Work out the finished part from the listing and answer in its coordinate system (mm). Give positions to 0.01 mm unless a question says otherwise; leave off trailing zeros. Order: outer loops, then holes, each group sorted by start corner. A loop starts at its lowest first (then second) coordinate and runs counter-clockwise, first axis right, second up. Notation, with made-up numbers: (-39, 65.25) - (-28, 65.25) arc R11 cw to (-28, 73.25) - close; hole circle Ø9 at (-0.5, 41). An arc over 180 degrees is marked (long way). Write each question's results on one line, items separated by ' | '.
Autodesk Inventor part; units mm, degrees
ref_plane "YZ Plane" through (0, 0, 0) normal (1, 0, 0) x (0, 1, 0)
ref_plane "XZ Plane" through (0, 0, 0) normal (0, 1, 0) x (-1, 0, 0)
ref_plane "XY Plane" through (0, 0, 0) normal (0, 0, 1) x (1, 0, 0)
sketch "Sketch2" plane through (0, 0, 0) normal (0, 0, 1) x (1, 0, 0)
  circle A0 centre (0, 0) radius 6.35
  line L0 (0, 0) -> (0, 11.35)
  line L1 (0, 11.35) -> (9.8294, 5.675)
  line L2 (9.8294, 5.675) -> (9.8294, -5.675)
  line L3 (9.8294, -5.675) -> (0, -11.35)
  line L4 (0, -11.35) -> (-9.8294, -5.675)
  line L5 (-9.8294, -5.675) -> (-9.8294, 5.675)
  line L6 (-9.8294, 5.675) -> (0, 11.35)
  dimension "d11" = 12.7
extrude "Extrusion2" add sketch "Sketch2" along normal blind 30
thread "Thread2"
chamfer "Chamfer2" distance 1 angle 45 18 edges at (4.9147, 8.5125, 30) (9.8294, 0, 30) (4.9147, -8.5125, 30) (-4.9147, -8.5125, 30) (-9.8294, 0, 30) (-4.9147, 8.5125, 30) (9.8294, 5.675, 15) (9.8294, -5.675, 15) (0, -11.35, 15) (-9.8294, -5.675, 15) (-9.8294, 5.675, 15) (0, 11.35, 15) (-4.9147, 8.5125, 0) (4.9147, 8.5125, 0) (9.8294, 0, 0) (4.9147, -8.5125, 0) (-4.9147, -8.5125, 0) (-9.8294, 0, 0)
properties part number "5302_Brass_Nut_0.5_20_Tx_Rx_Relative_Positioning_MPSv2_v1" material "Brass, Soft Yellow"
1. A cutting plane is placed at B-B, the plane x = 6. Write down the section's boundary in (y, z), then the cut area to 3 significant figures.
Answer list:
outline: (-7.89, 1) - (-6.73, 0) - (-2.08, 0) - (-2.08, 30) - (-6.73, 30) - (-7.89, 29) - close; (2.08, 0) - (6.73, 0) - (7.89, 1) - (7.89, 29) - (6.73, 30) - (2.08, 30) - close | area: 346 mm^2
2. Straight lines are drawn through the part: line 1 (X direction, y = 0, z = 18); line 2 (Y direction, x = 0, z = 23.75); line 3 (Y direction, x = -4.25, z = 14). For each, find the intervals that lie inside material, in ascending order. Write a range as [from, to].
Answer list:
line 1: [-9.83, -6.35], [6.35, 9.83] | line 2: [-10.85, -6.35], [6.35, 10.85] | line 3: [-8.9, -4.72], [4.72, 8.9]
3. A cutting plane is placed at A-A, the plane y = 0. Write down the section's boundary in (x, z).
Answer list:
outline: (-9.83, 1) - (-8.83, 0) - (-6.35, 0) - (-6.35, 30) - (-8.83, 30) - (-9.83, 29) - close; (6.35, 0) - (8.83, 0) - (9.83, 1) - (9.83, 29) - (8.83, 30) - (6.35, 30) - close
4. A cutting plane is placed at D-D, the plane y = 7. Write down the section's boundary in (x, z).
Answer list:
outline: (-7.53, 1) - (-5.53, 0) - (5.53, 0) - (7.53, 1) - (7.53, 29) - (5.53, 30) - (-5.53, 30) - (-7.53, 29) - close
5. Given P1, Ø11.5, axis at x = 0, y = 0, coming from the +Z side; P2, Ø5, axis at y = 8.5, z = 7.5, coming from the +X side; P3, Ø4, axis at x = -6, z = 13, coming from the -Y side; P4, Ø3, axis at x = -7, z = 3.5, coming from the +Y side, each flat-ended and moving along its own axis, determine where each tip first touches the part or whether it passes through.
Answer list:
P1: through | P2: x = 9.06 | P3: y = -9.04 | P4: y = 8.17
6. A cutting plane is placed at C-C, the plane z = 7.5. Write down the section's boundary in (x, y) (3 decimals).
Answer list:
outline: (-9.829, -4.675) - (-8.963, -6.175) - (-0.866, -10.85) - (0.866, -10.85) - (8.963, -6.175) - (9.829, -4.675) - (9.829, 4.675) - (8.963, 6.175) - (0.866, 10.85) - (-0.866, 10.85) - (-8.963, 6.175) - (-9.829, 4.675) - close; hole circle Ø12.7 at (0, 0)
